For this review, take the finished solid that the model builds, in its own axes (mm). Face numbers are marked on the shaded views. A direction names the side the tool comes from. Coordinates: 2 decimals unless noted, no trailing zeros. Write each loop counter-clockwise with the first axis right and the second up, starting at its lowest first coordinate (ties: lowest second). Pieces come first, ordered by that corner, then holes. Notation, with made-up numbers: M -4.5,-36.5 L 12.5,-36.5 A15 ccw 12.5,-19.5 Z; hole C 11.5,70 d11. An arc over 180 degrees is marked long. One line per question, with ' | ' between items.
Autodesk Inventor part; units mm, degrees
ref_plane "YZ Plane" through (0, 0, 0) normal (1, 0, 0) x (0, 1, 0)
ref_plane "XZ Plane" through (0, 0, 0) normal (0, 1, 0) x (-1, 0, 0)
ref_plane "XY Plane" through (0, 0, 0) normal (0, 0, 1) x (1, 0, 0)
sketch "Sketch1" plane through (0, 0, 0) normal (0, 0, 1) x (1, 0, 0)
  circle A0 centre (0, 0) radius 7
  circle A1 centre (0, 0) radius 5
  circle A2 centre (0, 0) radius 1
  line L0 (-9, 0) -> (9, 0)
  line L1 (9, 0) -> (9, -14)
  line L2 (9, -14) -> (-9, -14)
  line L3 (-9, -14) -> (-9, 0)
  dimension "d11" = 14
  dimension "d12" = 10
  dimension "d13" = 2
  dimension "d18" = 14
  dimension "d19" = 18
extrude "Extrusion1" add sketch "Sketch1" along normal blind 27 contours L0 L1 L2 L3 A0 | A0 L0 A1 | A1 L0 A2 | A2 L0 picked at (6.2655, -0.5584) picked at (3.6182, -0.3989) picked at (-0.2952, -0.1549)
sketch "Sketch3" plane through (0, 0, 0) normal (0, 0, -1) x (-1, 0, 0)
  line L0 (9, -14) -> (9, 0)
  line L1 (-9, -14) -> (9, -14)
  line L2 (9, -14) -> (9, 8)
  line L3 (9, 8) -> (-9, 8)
  line L4 (-9, 8) -> (-9, -14)
  dimension "d22" = 22
extrude "Extrusion6" add sketch "Sketch3" along normal blind 2.5
extrude "Extrusion5" cut sketch "Sketch1" along normal blind 30 contours L0 A1 A0 | A0 L0 A1 | L0 A2 A1 | A1 L0 A2 | L0 A2 | A2 L0
extrude "Extrusion7" cut sketch "Sketch1" against normal through all contours L0 A2 A1 | A1 L0 A2 | L0 A2 | A2 L0
fillet "Fillet1" radius 8 2 edges at (-9, 8, -1.25) (9, 8, -1.25)
sketch "Sketch4" plane through (9, -14, 27) normal (1, 0, 0) x (0, 0, -1)
  line L0 (0, 0) -> (29.5, 0)
  line L1 (11.75, 3.5) -> (17.75, 3.5)
  line L2 (17.75, 3.5) -> (17.75, 1)
  line L3 (17.75, 1) -> (11.75, 1)
  line L4 (11.75, 1) -> (11.75, 3.5)
  point P0 (14.75, 0)
  point P1 (14.75, 1)
  dimension "d32" = 6
  dimension "d33" = 2.5
  dimension "d34" = 1
extrude "Extrusion8" cut sketch "Sketch4" against normal through all
sketch "Sketch5" plane through (0, 0, -2.5) normal (0, 0, -1) x (-1, 0, 0)
  line L0 (9, -14) -> (9, 0)
  line L1 (-9, -14) -> (9, -14)
  line L2 (9, -14) -> (9, -6.5)
  line L3 (9, -6.5) -> (-9, -6.5)
  line L4 (-9, -6.5) -> (-9, -14)
  dimension "d37" = 7.5
extrude "Extrusion9" add sketch "Sketch5" along normal blind 33
sketch "Sketch6" plane through (-9, -6.5, -2.5) normal (0, 1, 0) x (1, 0, 0)
  line L0 (4.8, 10) -> (13.2, 10)
  line L1 (13.2, 10) -> (13.2, 33)
  line L2 (13.2, 33) -> (4.8, 33)
  line L3 (4.8, 33) -> (4.8, 10)
  line L4 (0, 33) -> (18, 33)
  point P0 (9, -2.5)
  point P1 (9, 33)
  point P2 (9, 33)
  dimension "d45" = 23
  dimension "d47" = 0
  dimension "d69" = 8.4
extrude "Extrusion10" cut sketch "Sketch6" against normal blind 30
sketch "Sketch7" plane through (9, -14, 27) normal (1, 0, 0) x (0, 0, -1)
  line L0 (42.5, 5.35) -> (60.5, 5.35)
  line L1 (60.5, 5.35) -> (60.5, 2.15)
  line L2 (60.5, 2.15) -> (42.5, 2.15)
  line L3 (42.5, 2.15) -> (42.5, 5.35)
  line L4 (62.5, 7.5) -> (62.5, 0)
  line L5 (62.5, 7.5) -> (39.5, 7.5)
  point P0 (27, 14)
  point P1 (60.5, 3.75)
  point P2 (62.5, 3.75)
  point P3 (51.5, 5.35)
  point P4 (51, 7.5)
  point P5 (59.5, 7.5)
  dimension "d49" = 3.2
  dimension "d55" = 18
  dimension "d70" = 20
extrude "Extrusion11" cut sketch "Sketch7" against normal through all
sketch "Sketch8" plane through (-9, -6.5, -2.5) normal (0, 1, 0) x (1, 0, 0)
  circle A0 centre (9, 4.5) radius 3
  circle A1 centre (9, -25.5) radius 3
  line L0 (16, -29.5) -> (2, -29.5)
  point P0 (9, -2.5)
  dimension "d56" = 6
  dimension "d57" = 6
  dimension "d58" = 4
  dimension "d59" = 34
extrude "Extrusion12" cut sketch "Sketch8" along normal mid plane 10
sketch "Sketch9" plane through (0, -11.5, -7) normal (0, 1, 0) x (1, 0, 0)
  circle A0 centre (0, 0) radius 3
  circle A1 centre (0, 0) radius 1.6
  circle A2 centre (0, -30) radius 1.6
  point P0 (0, -7)
  dimension "d62" = 3.2
  dimension "d63" = 3.2
extrude "Extrusion13" cut sketch "Sketch9" against normal through all contours A1 | A2
chamfer "Chamfer2" distance 2.2 angle 45 4 edges at (4.2, -6.5, -24) (-4.2, -6.5, -24) (6.6, -6.5, -35.5) (-6.6, -6.5, -35.5)
properties part number "Solinoid holder"
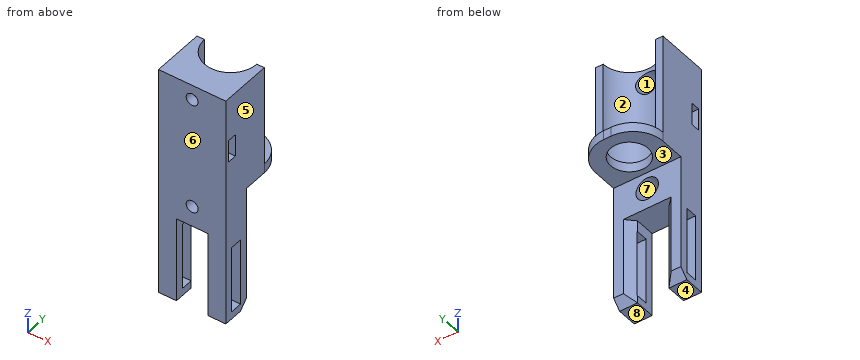
1. Take a section at B-B on x = 0. Give the number of separate pieces and of enclosed holes in the cut face, plus the area to 3 significant figures.
Computed values:
separate pieces: 4 | enclosed holes: 1 | area: 206 mm2
2. Take a section at A-A on z = 11. State the section outline as (x, y) points.
Computed values:
outline: M -9,-14 L 9,-14 L 9,-13 L -9,-13 Z; M -9,-10.5 L 9,-10.5 L 9,0 L 7,0 A7 cw -7,0 L -9,0 Z
3. Machinability: for the marked faces 1, 2, 3, 4 and 5, which of the approach directions +Z, -Z, +X, -X, +Y, -Y give a long, thin tool a straight path to every point of the face, cutting with its end or side? Answer none if there is none.
Computed values:
face 1: +Y | face 2: +Z, +Y | face 3: -Z, +X, -X, +Y | face 4: -Z, +X, -X, +Y, -Y | face 5: +Z, -Z, +X, +Y, -Y
4. Draft analysis for pull direction Z (two halves, no side actions). For the marked faces 6, 7 and 8, state which applies: pulls with the +Z half, pulls with the -Z half, needs draft (parallel to the pull), parting line crosses it, or undercut.
Computed values:
face 6: needs draft | face 7: undercut | face 8: pulls with the -Z half
5. Take a section at D-D on z = -19. State the section outline as (x, y) points, plus the area to 3 significant figures.
Computed values:
outline: M -9,-14 L -4.2,-14 L -4.2,-11.85 L -9,-11.85 Z; M -9,-8.65 L -4.25,-8.65 L -6.4,-6.5 L -9,-6.5 Z; M 4.2,-14 L 9,-14 L 9,-11.85 L 4.2,-11.85 Z; M 4.25,-8.65 L 9,-8.65 L 9,-6.5 L 6.4,-6.5 Z | area: 36.4 mm2
6. Take a section at C-C on y = 2.75. State the section outline as (x, z) points.
Computed values:
outline: M -8.51,-2.5 L -4.18,-2.5 L -4.18,0 L -8.51,0 Z; M 4.18,-2.5 L 8.51,-2.5 L 8.51,0 L 4.18,0 Z
7. For line 1 along Z through (x, y) = (0, -9.55); line 2 along Z through (x, y) = (0, -13.45); line 3 along Z through (x, y) = (0, -12.1), list the stretches that pass through material, from the lowest coordinate up.
Computed values:
line 1: z = -12.5 to -10, -4 to 20, 26 to 27 | line 2: z = -12.5 to -8.6, -5.4 to 21.4, 24.6 to 27 | line 3: z = -12.5 to -8.6, -5.4 to 9.25, 15.25 to 21.4, 24.6 to 27
8. Clearance check with flat-ended pins moving along their axes: P1, Ø8, axis at x = 0, z = 23, coming from the -Y side; P2, Ø1, axis at x = 3.5, z = -26.5, coming from the -Y side; P3, Ø4, axis at x = 1, y = -9, coming from the -Z side; P4, Ø6.5, axis at x = 0, z = -6, coming from the +Y side. State where each tip first meets the part, or that it passes through.
Computed values:
P1: stops at y = -14 | P2: passes through | P3: stops at z = -12.5 | P4: stops at y = -6.5
